```python
from build123d import *

# Parameters (mm, degrees)
SKETCH1_W           = 25.4
SKETCH1_H           = 50.8
SKETCH1_W_2         = 20.32
SKETCH1_H_2         = 45.72
EXTRUDE_THIN1_DEPTH = 381
SKETCH2_R           = 2.0701
CUT_EXTRUDE1_DEPTH  = 51.8
LPATTERN1_COUNT     = 31
LPATTERN1_PITCH     = 25.4
SKETCH3_R           = 19.05
SKETCH3_R_2         = 3.175
SKETCH3_R_3         = 2.413
SKETCH3_R_4         = 2.54
CUT_EXTRUDE2_DEPTH  = 26.4
SKETCH3_3_R         = 2.0193
CUT_EXTRUDE3_DEPTH  = 26.4


with BuildPart() as part:
    # Sketch1 → Extrude-Thin1 (new body, symmetric)
    with BuildSketch(Plane.XY):
        Rectangle(SKETCH1_W, SKETCH1_H)
        Rectangle(SKETCH1_W_2, SKETCH1_H_2, mode=Mode.SUBTRACT)
    extrude(amount=EXTRUDE_THIN1_DEPTH, both=True)

    # Sketch2 → Cut-Extrude1 (cut, through all)
    with BuildSketch(Plane(origin=(0, 25.4, 0), x_dir=(1, 0, 0), z_dir=(0, 1, 0))):
        with Locations((0, -368.3)):
            Circle(SKETCH2_R)
    cut_extrude1 = extrude(amount=-CUT_EXTRUDE1_DEPTH, mode=Mode.SUBTRACT)

    # LPattern1: Cut-Extrude1 ×31
    with Locations(*[(0, 0, -i * LPATTERN1_PITCH) for i in range(1, LPATTERN1_COUNT)]):
        add(cut_extrude1, mode=Mode.SUBTRACT)

    # Sketch3 → Cut-Extrude2 (cut, through all)
    with BuildSketch(Plane(origin=(12.7, 0, 0), x_dir=(0, 0, -1), z_dir=(1, 0, 0))):
        with Locations((0, -3.175)):
            Circle(SKETCH3_R)
        with Locations((-23.8125, -3.175)):
            Circle(SKETCH3_R_2)
        with Locations((-57.0865, -3.175)):
            Circle(SKETCH3_R_3)
        with Locations((-35.4965, 14.605)):
            Circle(SKETCH3_R_4)
        with Locations((23.8125, -3.175)):
            Circle(SKETCH3_R_2)
        with Locations((35.4965, 14.605)):
            Circle(SKETCH3_R_4)
        with Locations((57.0865, -3.175)):
            Circle(SKETCH3_R_3)
    extrude(amount=-CUT_EXTRUDE2_DEPTH, mode=Mode.SUBTRACT)

    # Sketch3<3> → Cut-Extrude3 (cut, through all)
    with BuildSketch(Plane(origin=(12.7, 0, 0), x_dir=(0, 0, -1), z_dir=(1, 0, 0))):
        with BuildLine():
            Line((-275.571100521, -9.525), (-264.141100521, -9.525))
            ThreePointArc((-264.141100521, -9.525), (-254.616100521, 0), (-264.141100521, 9.525))
            Line((-264.141100521, 9.525), (-275.571100521, 9.525))
            ThreePointArc((-275.571100521, 9.525), (-285.096100521, 0), (-275.571100521, -9.525))
        make_face()
        with Locations((-220.961100521, 0)):
            Circle(SKETCH3_3_R)
    cut_extrude3 = extrude(amount=-CUT_EXTRUDE3_DEPTH, mode=Mode.SUBTRACT)

    # Mirror1: Cut-Extrude3 across plane
    add(cut_extrude3.mirror(Plane.XY), mode=Mode.SUBTRACT)


solid = part.part
```
Work out the finished part from the listing and answer in its coordinate system (mm). A direction names the side the tool comes from. Coordinates: 2 decimals unless noted, no trailing zeros. Order: outer loops, then holes, each group sorted by start corner. A loop starts at its lowest first (then second) coordinate and runs counter-clockwise, first axis right, second up. Notation, with made-up numbers: (15, 61) - (71, 61) arc R38 ccw to (71, 99) - close; hole circle Ø3 at (83, -32.5). An arc over 180 degrees is marked (long way). Answer as a JSON object with one key per item and string values.
1. Find section A-A on z = -204.5. Determine the outline of the cut face in (x, y), plus the area to 3 significant figures.
Output values:
{"outline": "(-12.7, -25.4) - (12.7, -25.4) - (12.7, 25.4) - (-12.7, 25.4) - close; hole (-10.16, -22.86) - (10.16, -22.86) - (10.16, 22.86) - (-10.16, 22.86) - close", "area": "361 mm²"}
2. Consider line 1 (Y direction, x = 3.75, z = 189.5); line 2 (X direction, y = 14.5, z = -236); line 3 (X direction, y = -24, z = 368). Determine where each line is inside the solid, lowest interval first.
Output values:
{"line 1": "y = -25.4 to -22.86, 22.86 to 25.4", "line 2": "x = -12.7 to -10.16, 10.16 to 12.7", "line 3": "x = -12.7 to -2.05, 2.05 to 12.7"}
3. This flat-tipped pin is pushed along its axis until it touches: P1, Ø3.5, axis at x = 0, z = -190.5, coming from the +Y side. Where does it stop, or does it pass through?
Output values:
{"P1": "passes through"}
4. The mould has two halves that part along X. Classify faces 3 (the face through (-10.4, 2, -381)), 4 (the face through (-10.16, 20, 5)), 5 (the face through (-12.7, 17, 5)), 6 (the face through (10.16, 20, 5)): +X half, -X half, draft (parallel to the pull), parting line (faces both ways), or undercut.
Output values:
{"face 3": "draft", "face 4": "undercut", "face 5": "-X half", "face 6": "undercut"}
5. A tool of negligible diameter and unlimited length cuts with its end or side. For faces 1 (the face through (0, -22.86, 5)), 2 (the face through (0, -25.4, 5)), from which of +Z, -Z, +X, -X, +Y, -Y can it reach the whole face along a straight path? Write none if from no direction.
Output values:
{"face 1": "+Z, -Z", "face 2": "+Z, -Z, +X, -X, -Y"}
